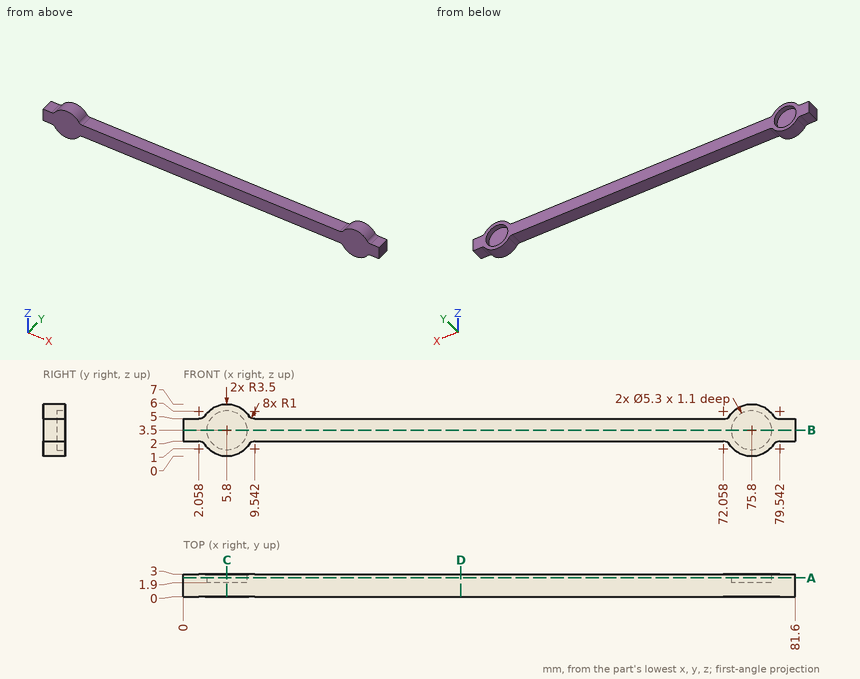
Design review of the part shown in the three views and the two pictorial views. Dimensions are in mm from the part's minimum x, y and z. Coordinates: 2 decimals unless noted, no trailing zeros. Write each loop counter-clockwise with the first axis right and the second up, starting at its lowest first coordinate (ties: lowest second). Pieces come first, ordered by that corner, then holes. Notation, with made-up numbers: (8.25, 50.5) - (21.25, 50.5) arc R5 cw to (21.25, 58.5) - close; hole circle Ø7 at (61.25, -36). An arc over 180 degrees is marked (long way). Write item = value, one per line.
(1) Consider section A-A, the plane y = 2.55. State how many separate pieces and enclosed holes the cut face has.
Result sheet:
separate_pieces = 1
enclosed_holes = 2
(2) Consider section B-B, the plane z = 3.5. Give the boundary of the cut face in (x, y), then the cut area to 3 significant figures.
Result sheet:
outline = (0, 0) - (81.6, 0) - (81.6, 3) - (78.45, 3) - (78.45, 1.9) - (73.15, 1.9) - (73.15, 3) - (8.45, 3) - (8.45, 1.9) - (3.15, 1.9) - (3.15, 3) - (0, 3) - close
area = 233 mm^2
(3) Consider section C-C, the plane x = 5.8. Give the boundary of the cut face in (y, z).
Result sheet:
outline = (0, 0) - (3, 0) - (3, 0.85) - (1.9, 0.85) - (1.9, 6.15) - (3, 6.15) - (3, 7) - (0, 7) - close
(4) For P1, Ø1, axis at x = 15, y = 2.5, coming from the -Z side; P2, Ø1, axis at x = 64.5, y = 2.5, coming from the +Z side; P3, Ø2.5, axis at x = 76.5, z = 2.5, coming from the +Y side, all flat-tipped, find the tip position at first contact; note any pin that passes through.
Result sheet:
P1 = 2
P2 = 5
P3 = 1.9
(5) For line 1 (X direction, y = 2.3, z = 3.5); line 2 (Z direction, x = 75.8, y = 2.2); line 3 (X direction, y = 2.1, z = 4.25), list the stretches that pass through material, from the lowest coordinate up. Write a range as [from, to].
Result sheet:
line_1 = [0, 3.15], [8.45, 73.15], [78.45, 81.6]
line_2 = [0, 0.85], [6.15, 7]
line_3 = [0, 3.26], [8.34, 73.26], [78.34, 81.6]
(6) Consider section D-D, the plane x = 37. Give the boundary of the cut face in (y, z).
Result sheet:
outline = (0, 2) - (3, 2) - (3, 5) - (0, 5) - close
